Autodesk Inventor part; units mm, degrees
ref_plane "YZ Plane" through (0, 0, 0) normal (1, 0, 0) x (0, 1, 0)
ref_plane "XZ Plane" through (0, 0, 0) normal (0, 1, 0) x (-1, 0, 0)
ref_plane "XY Plane" through (0, 0, 0) normal (0, 0, 1) x (1, 0, 0)
sketch "Sketch1" plane through (0, 0, 0) normal (1, 0, 0) x (0, 1, 0)
  line L0 (50, 41.5) -> (-50, 41.5)
  line L1 (-50, 41.5) -> (-50, -41.5)
  line L2 (-50, -41.5) -> (50, -41.5)
  line L3 (50, -41.5) -> (50, 41.5)
  point P0 (0, 0)
  point P1 (50, 0)
  point P2 (0, -41.5)
  dimension "d0" = 100
  dimension "d1" = 83
extrude "Extrusion1" add sketch "Sketch1" along normal blind 1.6
sketch "Sketch12" plane through (0, 50, 41.5) normal (0, 1, 0) x (1, 0, 0)
  line L0 (0, 83) -> (0, 0)
  line L1 (0, 0) -> (1.6, 0)
  line L2 (1.6, 83) -> (1.6, 0)
  line L3 (0, 83) -> (1.6, 83)
  point P0 (0, 41.5)
extrude "Extrusion3" add sketch "Sketch12" along normal blind 56.75
sketch "Sketch13" plane through (0, -50, -41.5) normal (0, -1, 0) x (1, 0, 0)
  line L0 (0, 83) -> (0, 0)
  line L1 (0, 0) -> (1.6, 0)
  line L2 (1.6, 83) -> (1.6, 0)
  line L3 (0, 83) -> (1.6, 83)
  point P0 (0, 41.5)
extrude "Extrusion4" add sketch "Sketch13" along normal blind 56.75
sketch "Sketch14" plane through (0, 0, 0) normal (-1, 0, 0) x (0, 0, 1)
  point P0 (0, 0)
  point P1 (27.5, -51.25)
  point P2 (27.5, 51.25)
  point P3 (-27.5, -51.25)
  point P4 (-27.5, 51.25)
  dimension "d156" = 102.5
  dimension "d157" = 102.5
  dimension "d158" = 55
  dimension "d159" = 27.5
  dimension "d160" = 51.25
hole "Hole7" at (0, -51.25, 27.5) at (0, 51.25, 27.5) at (0, -51.25, -27.5) at (0, 51.25, -27.5) direction (1, 0, 0) diameter 6 end through all
sketch "Sketch16" plane through (0, 0, 0) normal (-1, 0, 0) x (0, 0, 1)
  circle A0 centre (-27.5, -51.25) radius 3
  circle A1 centre (27.5, -51.25) radius 3
  circle A2 centre (27.5, 51.25) radius 3
  circle A3 centre (-27.5, 51.25) radius 3
  line L0 (41.5, -106.75) -> (41.5, 106.75)
  line L1 (-41.5, 106.75) -> (41.5, 106.75)
  line L2 (-41.5, 106.75) -> (-41.5, -106.75)
  line L3 (41.5, -106.75) -> (-41.5, -106.75)
  line L4 (0, 0) -> (-25, 0) construction
  point P0 (35, -100.75)
  point P1 (-35, -100.75)
  point P2 (35, 100.75)
  point P3 (-35, 100.75)
  dimension "d168" = 70
  dimension "d169" = 6
  dimension "d170" = 35
hole "Hole8" at (0, -100.75, 35) at (0, -100.75, -35) at (0, 100.75, 35) at (0, 100.75, -35) direction (1, 0, 0) diameter 6 end through all
sketch "Sketch19" plane through (0, 0, 0) normal (-1, 0, 0) x (0, 0, 1)
  circle A0 centre (-27.5, 51.25) radius 3 construction
  line L0 (-39, 76.75) -> (-39, 72) construction
  line L1 (-39, 76.75) -> (-39, 81.5) construction
  line L2 (-41.5, 106.75) -> (-41.5, -106.75) construction
  line L3 (-41.5, 106.75) -> (41.5, 106.75)
  point P0 (0, 0)
  dimension "d194" = 4.75
  dimension "d195" = 4.75
  dimension "d203" = 25.25
  dimension "d204" = 2.5
hole "Hole9" at (0, 72, -39) at (0, 81.5, -39) direction (1, 0, 0) diameter 2.6 end through all
sketch "Sketch21" plane through (0, 0, 0) normal (-1, 0, 0) x (0, 0, 1)
  line L0 (-41.5, 106.75) -> (-41.5, -106.75)
  line L1 (-41.5, 85.75) -> (-36.5, 85.75)
  line L2 (-36.5, 85.75) -> (-36.5, 67.75)
  line L3 (-36.5, 67.75) -> (-41.5, 67.75)
  line L4 (-41.5, 67.75) -> (-41.5, 85.75)
  line L5 (-41.5, 106.75) -> (41.5, 106.75)
  point P0 (0, 0)
  point P1 (-41.5, 67.75)
  dimension "d205" = 5
  dimension "d206" = 21
  dimension "d207" = 18
extrude "Extrusion5" cut sketch "Sketch21" against normal through all
sketch "Sketch23" plane through (0, 0, 0) normal (-1, 0, 0) x (0, 0, 1)
  circle A0 centre (-35, 100.75) radius 3
  line L0 (0, 0) -> (-12.2775, 0) construction
  point P0 (38, 93.75)
  point P1 (-38, 93.75)
  point P2 (38, -93.75)
  point P3 (-38, -93.75)
  dimension "d220" = 76
  dimension "d221" = 38
  dimension "d229" = 7
hole "Hole11" at (0, 93.75, 38) at (0, 93.75, -38) at (0, -93.75, 38) at (0, -93.75, -38) direction (1, 0, 0) diameter 3.454 end through all
equation "\"d195\" = d194"
properties part number "SolarPCB_RBF_EGSE" material "Acetal Resin, Black"
Source: CAD feature listing. Evaluate the final solid. Frame: model axes, mm. Give positions to 0.01 mm unless a question says otherwise; leave off trailing zeros. Write each loop counter-clockwise with the first axis right and the second up, starting at its lowest first coordinate (ties: lowest second). Pieces come first, ordered by that corner, then holes. Notation, with made-up numbers: (-3, 36.25) -> (35, 36.25) arc R12 cw to (35, 59.25) -> close; hole circle Ø8 at (-4.75, -39). An arc over 180 degrees is marked (long way). Write item = value, one per line.
Q1. Cut plane C-C on x = 0.4. State how many separate pieces and enclosed holes the cut face has, then the cut area to 3 significant figures.
Here are the results:
separate_pieces = 1
enclosed_holes = 12
area = 17,400 mm²
Q2. Line query: line 1 (Z direction, x = 0.55, y = 51.25); line 2 (Y direction, x = 0.75, z = -35); line 3 (Z direction, x = 1.25, y = 100.75). Output: solid intervals per line, ascending. Write a range as from..to.
Here are the results:
line_1 = -41.5..-30.5, -24.5..24.5, 30.5..41.5
line_2 = -106.75..-103.75, -97.75..97.75, 103.75..106.75
line_3 = -41.5..-38, -32..32, 38..41.5
Q3. Mould query, pull axis Y, two halves, no side actions, for faces 1 (the face through (0.811, -95.206, 38.928)), 2 (the face through (0, 1, 1)), 3 (the face through (0.81, -97.82, 34.35)). Classes: +Y half, -Y half, draft (parallel to the pull), parting line (faces both ways), or undercut.
Here are the results:
face_1 = undercut
face_2 = draft
face_3 = undercut
Q4. Cut plane A-A on z = -27.5. Return loops of the section in (x, y), then the cut area to 3 significant figures.
Here are the results:
outline = (0, -106.75) -> (1.6, -106.75) -> (1.6, -54.25) -> (0, -54.25) -> close; (0, -48.25) -> (1.6, -48.25) -> (1.6, 48.25) -> (0, 48.25) -> close; (0, 54.25) -> (1.6, 54.25) -> (1.6, 106.75) -> (0, 106.75) -> close
area = 322 mm²
Q5. Cut plane B-B on y = 51.25. Return loops of the section in (x, z), then the cut area to 3 significant figures.
Here are the results:
outline = (0, -41.5) -> (1.6, -41.5) -> (1.6, -30.5) -> (0, -30.5) -> close; (0, -24.5) -> (1.6, -24.5) -> (1.6, 24.5) -> (0, 24.5) -> close; (0, 30.5) -> (1.6, 30.5) -> (1.6, 41.5) -> (0, 41.5) -> close
area = 114 mm²
Q6. First-contact query: pin 1 (0.5 mm diameter, centred on x = 1, y = 79, fed in from -Z). Flat tip, straight axial feed; report the tip coordinate or a pass-through.
Here are the results:
pin_1 = -36.5
